Read the model definition and answer for the solid it produces. Units are mm, in the model's axes. A direction names the side the tool comes from. Coordinates: 2 decimals unless noted, no trailing zeros. Loops run counter-clockwise (first coordinate to the right, second up) from the corner with the lowest first, then second, coordinate; pieces in that order, holes last. Notation, with made-up numbers: (-39, 80) - (-14, 80) arc R13 ccw to (-14, 91) - close; hole circle Ø3 at (-20.75, 86). An arc over 180 degrees is marked (long way). Use one line per item in the form item = value. Start each with the question number.
1) Each of these flat-tipped pins is pushed along its axis until it touches: P1, Ø8, axis at y = 0, z = 0, coming from the +X side; P2, Ø2, axis at y = -6, z = 10, coming from the -X side; P3, Ø1.6, axis at y = -5.62, z = -9.74, coming from the -X side. Where does it stop, or does it pass through?
2) A cutting plane is placed at A-A (y = 0). Give the vertices of the cut face in (x, z), and give its area (3 significant figures).
3) The mould has two halves that part along Y. Classify faces 4 (the face through (22.77, -10.26, -0.13)), 5 (the face through (22.77, 10.36, 0.46)), 6 (the face through (9.633, -3.966, 0.521)), 7 (the face through (6, 3, 0)): released by +Y, released by -Y, zero draft, split by the parting line, or undercut.
4) Which of the six approach directions +Z, -Z, +X, -X, +Y, -Y give full straight-line access (tool end or side, diameter ignored) to faces 1 (the face through (54.1, 0, 0)), 2 (the face through (65.1, 0, -6)), 3 (the face through (24.6, -11, 0))?
5) A cutting plane is placed at D-D (x = 41). Give the vertices of the cut face in (y, z), and give its area (3 significant figures).
6) A cutting plane is placed at C-C (x = 55.5). Give the vertices of the cut face in (y, z), and give its area (3 significant figures).
7) Consider line 1 (Y direction, x = 22.5, z = 0); line 2 (Y direction, x = 64, z = 0); line 3 (Z direction, x = 24, y = 5.5). Determine where each line is inside the solid, lowest interval first.
from build123d import *

# Parameters (mm, degrees)
SZKIC2_R                   = 1
WYTNIJ_WYCI_GNI_CIE1_DEPTH = 3.6
WYTNIJ_WYCI_GNI_CIE2_START = -12
WYTNIJ_WYCI_GNI_CIE2_DEPTH = 12


with BuildPart() as part:
    # Szkic1 → Obrót1 (revolve)
    with BuildSketch(Plane.XY, mode=Mode.PRIVATE) as obr_t1_sk:
        Polygon((0, 0), (0, 4), (19, 4), (19, 9.5), (21, 9.5), (21, 13), (65.1, 13), (65.1, 5), (61.85, 5), (61.85, 1.5), (54.1, 1.5), (54.1, 0), align=None)
    revolve(obr_t1_sk.sketch.rotate(Axis((0, 0, 0), (-1, 0, 0)), 90), axis=Axis((0, 0, 0), (-1, 0, 0)))

    # Szkic2 → Wytnij-wyciągnięcie1 (cut)
    with BuildSketch(Plane.ZY.offset(-21)):
        with Locations((0, 11.25)):
            Circle(SZKIC2_R)
        with Locations((9.742785793, 5.625)):
            Circle(SZKIC2_R)
        with Locations((9.742785793, -5.625)):
            Circle(SZKIC2_R)
        with Locations((0, -11.25)):
            Circle(SZKIC2_R)
        with Locations((-9.742785793, -5.625)):
            Circle(SZKIC2_R)
        with Locations((-9.742785793, 5.625)):
            Circle(SZKIC2_R)
    extrude(amount=-WYTNIJ_WYCI_GNI_CIE1_DEPTH, mode=Mode.SUBTRACT)

    # Szkic3 → Wytnij-wyciągnięcie2 (cut)
    with BuildSketch(Plane.ZY.offset(WYTNIJ_WYCI_GNI_CIE2_START)):
        with BuildLine():
            Line((-2.645751311, 3), (2.645751311, 3))
            ThreePointArc((2.645751311, 3), (0, 4), (-2.645751311, 3))
        make_face()
    extrude(amount=WYTNIJ_WYCI_GNI_CIE2_DEPTH, mode=Mode.SUBTRACT)


solid = part.part
Found:
q1.P1 = 61.85
q1.P2 = 21
q1.P3 = 24.6
q2.outline = (0, -4) - (19, -4) - (19, -9.5) - (21, -9.5) - (21, -13) - (65.1, -13) - (65.1, -5) - (61.85, -5) - (61.85, -1.5) - (54.1, -1.5) - (54.1, 1.5) - (61.85, 1.5) - (61.85, 5) - (65.1, 5) - (65.1, 13) - (21, 13) - (21, 9.5) - (19, 9.5) - (19, 4) - (0, 4) - close
q2.area = 1,280 mm^2
q3.face_4 = undercut
q3.face_5 = undercut
q3.face_6 = split by the parting line
q3.face_7 = released by +Y
q4.face_1 = +X
q4.face_2 = +Z, -Z, +X, +Y, -Y
q4.face_3 = -X
q5.outline = circle Ø26 at (0, 0)
q5.area = 531 mm^2
q6.outline = circle Ø26 at (0, 0); hole circle Ø3 at (0, 0)
q6.area = 524 mm^2
q7.line_1 = -13 to -12.25, -10.25 to 10.25, 12.25 to 13
q7.line_2 = -13 to -5, 5 to 13
q7.line_3 = -11.78 to -10.73, -8.75 to 8.75, 10.73 to 11.78
